```python
from build123d import *

# Parameters (mm, degrees)
SKETCH_2_W      = 36
SKETCH_2_H      = 36
EXTRUDE_1_DEPTH = 11.2
SKETCH_3_W      = 25
SKETCH_3_H      = 25
EXTRUDE_2_DEPTH = 3.8
SKETCH_4_R      = 7
EXTRUDE_3_DEPTH = 7.6


with BuildPart() as part:
    # 草图2 → 凸台-拉伸1 (new body)
    with BuildSketch(Plane.XY):
        Rectangle(SKETCH_2_W, SKETCH_2_H)
    extrude(amount=EXTRUDE_1_DEPTH)

    # 草图3 → 凸台-拉伸2 (add)
    with BuildSketch(Plane.XY.offset(11.2)):
        Rectangle(SKETCH_3_W, SKETCH_3_H)
    extrude(amount=EXTRUDE_2_DEPTH)

    # 草图4 → 凸台-拉伸3 (add)
    with BuildSketch(Plane.XY.offset(15)):
        with Locations(Location((0, 0, 0), (0, 0, 180))):
            Circle(SKETCH_4_R)
    extrude(amount=EXTRUDE_3_DEPTH)

    # 草图6 → M3 螺纹孔1 (revolve, cut)
    with BuildSketch(Plane(origin=(-18, 0, 5.6), x_dir=(0, 0, 1), z_dir=(0, 1, 0))):
        Polygon((0, 0), (0, 8.251075774), (1.25, 7.5), (1.25, 6), (1.5, 6), (1.5, 0), align=None)
    hole_wizard_m3_1 = revolve(axis=Axis((-24.35, 0, 5.6), (1, 0, 0)), mode=Mode.SUBTRACT)

    # 镜向1: M3 螺纹孔1 across plane
    add(hole_wizard_m3_1.mirror(Plane(origin=(0, 0, 0), x_dir=(0, 0, 1), z_dir=(1, 0, 0))), mode=Mode.SUBTRACT)


solid = part.part
```
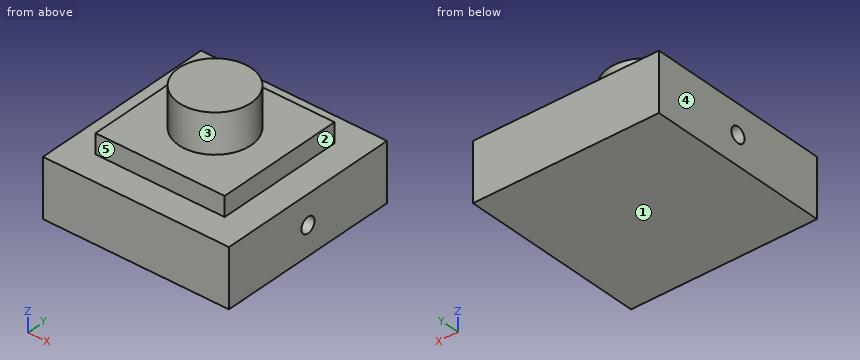
Geometry check sheet. Reference: the model listing, model coordinates, mm. Face numbers are marked on the shaded views. A direction names the side the tool comes from. Round coordinates to 2 decimals unless told otherwise and drop trailing zeros. Order: outer loops, then holes, each group sorted by start corner. A loop starts at its lowest first (then second) coordinate and runs counter-clockwise, first axis right, second up. Notation, with made-up numbers: (80.25, -5.75) - (123.25, -5.75) arc R30 cw to (123.25, 17.25) - close; hole circle Ø11 at (67, 6). An arc over 180 degrees is marked (long way). Use a Markdown table: item, result. Add a question column.
1) Section check D-D (z = 13). Record the cut outline in (x, y).
2) Thickness scan on line 1 along Z through (x, y) = (16, 0); line 2 along Y through (x, z) = (14.15, 5.6); line 3 along Y through (x, z) = (-10.9, 5.6). Record the ranges inside material, lowest first.
3) Section check B-B (x = -8). Record the cut outline in (y, z).
4) Set-up check for the marked faces 1, 2, 3, 4 and 5: record each of +Z, -Z, +X, -X, +Y, -Y from which the full face is reachable in a straight line by a thin tool's end or side.
5) Gauge pin test, flat ends, axial feed: P1, Ø12, axis at x = 13.5, z = 17, coming from the +Y side; P2, Ø4, axis at x = -4.5, z = 15.5, coming from the -Y side; P3, Ø1.8, axis at y = 0, z = 5.6, coming from the +X side; P4, Ø1.1, axis at y = -6, z = 13, coming from the +X side. Record the tip position at first contact, or that the pin passes through.
6) Section check A-A (x = 11). Record the cut outline in (y, z), then the cut area to 3 significant figures.
Established:
| question | item | result |
|---|---|---|
| 1 | outline | (-12.5, -12.5) - (12.5, -12.5) - (12.5, 12.5) - (-12.5, 12.5) - close |
| 2 | line 1 | 0 to 4.1, 7.1 to 11.2 |
| 2 | line 2 | -18 to -1.5, 1.5 to 18 |
| 2 | line 3 | -18 to -1.25, 1.25 to 18 |
| 3 | outline | (-18, 0) - (18, 0) - (18, 11.2) - (12.5, 11.2) - (12.5, 15) - (-12.5, 15) - (-12.5, 11.2) - (-18, 11.2) - close |
| 4 | face 1 | -Z, +X, -X, +Y, -Y |
| 4 | face 2 | +Z, +X, +Y, -Y |
| 4 | face 3 | +Z |
| 4 | face 4 | +Z, -Z, -X, +Y, -Y |
| 4 | face 5 | +Z, +X, -X, -Y |
| 5 | P1 | y = 18 |
| 5 | P2 | y = -12.5 |
| 5 | P3 | x = 10.29 |
| 5 | P4 | x = 12.5 |
| 6 | outline | (-18, 0) - (18, 0) - (18, 11.2) - (12.5, 11.2) - (12.5, 15) - (-12.5, 15) - (-12.5, 11.2) - (-18, 11.2) - close; hole circle Ø2.5 at (0, 5.6) |
| 6 | area | 493 mm2 |
